Could you check a few things on this model? Use its own coordinates, in mm. A direction names the side the tool comes from. Coordinates: 2 decimals unless noted, no trailing zeros. Loops run counter-clockwise (first coordinate to the right, second up) from the corner with the lowest first, then second, coordinate; pieces in that order, holes last. Notation, with made-up numbers: (55.5, -39.75) -> (87.5, -39.75) arc R28 ccw to (87.5, -8.75) -> close; hole circle Ø2 at (17, 38.25). An arc over 180 degrees is marked (long way). One line per question, with ' | ' between items.
from build123d import *

# Parameters (mm, degrees)
F1_DEPTH = 4
F0_R     = 1.5
F2_DEPTH = 1


with BuildPart() as f1:
    # F0 (on Top) → F1 (new body)
    with BuildSketch(Plane.XY):
        Polygon((11.5, 35.8), (-11.5, 35.8), (-11.5, -35.8), (11.5, -35.8), (11.5, -34.45), (-10.15, -34.45), (-10.15, 34.45), (11.5, 34.45), align=None)
    extrude(amount=F1_DEPTH)

    # F0 (on Top) → F2 (join)
    with BuildSketch(Plane.XY):
        Polygon((11.5, 5), (11.5, 34.45), (-10.15, 34.45), (-10.15, -34.45), (11.5, -34.45), (11.5, -5), (18.5, -5), (18.5, 5), align=None)
        with Locations((15, 0)):
            Circle(F0_R, mode=Mode.SUBTRACT)
    extrude(amount=F2_DEPTH)


solid = f1.part
1) We'd pull the mould along X, two halves only. Please class faces 4 (the face through (-10.15, 0, 2)), 5 (the face through (0, 35.8, 2)), 6 (the face through (13.5, 0.07, 0.49)): pulls with the +X half, pulls with the -X half, needs draft (parallel to the pull), parting line crosses it, or undercut.
Data:
face 4: pulls with the +X half | face 5: needs draft | face 6: undercut
2) On a 3-axis mill with a long thin cutter (end or side, diameter ignored), from which of +Z, -Z, +X, -X, +Y, -Y can I reach the whole of each face in a straight line? I mean faces 1 (the face through (11.5, 21.5, 0.7)), 2 (the face through (11.5, -21.6, 0.8)), 3 (the face through (1, -34.45, 2)). Say none if no direction works.
Data:
face 1: +Z, -Z, +X, +Y | face 2: +Z, -Z, +X, -Y | face 3: +Z, +X
3) I need wall thicknesses on line 1 along Y through (x, z) = (15, 0.8); line 2 along Y through (x, z) = (-1.75, 2.9); line 3 along Z through (x, y) = (-1, -22.5). Which ranges of each line are inside material? Lowest first, please. Write a range as from..to.
Data:
line 1: -5..-1.5, 1.5..5 | line 2: -35.8..-34.45, 34.45..35.8 | line 3: 0..1
4) If we section it at B-B on x = 15: Please give me the cut outline in (y, z).
Data:
outline: (-5, 0) -> (-1.5, 0) -> (-1.5, 1) -> (-5, 1) -> close; (1.5, 0) -> (5, 0) -> (5, 1) -> (1.5, 1) -> close
5) If we section it at C-C on x = 7: Please give me the cut outline in (y, z), and give its area (3 significant figures).
Data:
outline: (-35.8, 0) -> (35.8, 0) -> (35.8, 4) -> (34.45, 4) -> (34.45, 1) -> (-34.45, 1) -> (-34.45, 4) -> (-35.8, 4) -> close | area: 79.7 mm²
6) I'm going to push flat-ended pins straight in: pin 1 Ø2.5 at (x, y) = (15, 0) entering from -Z; pin 2 Ø0.5 at (x, z) = (14, 0.5) entering from -Y; pin 3 Ø0.9 at (y, z) = (-4.5, 3) entering from +X; pin 4 Ø0.8 at (x, z) = (16.5, 0.5) entering from +Y. Where does each tip first touch, or does it pass through?
Data:
pin 1: through | pin 2: y = -5 | pin 3: x = -10.15 | pin 4: y = 5
7) If we section it at D-D on z = 1.65: Please give me the cut outline in (x, y), and give its area (3 significant figures).
Data:
outline: (-11.5, -35.8) -> (11.5, -35.8) -> (11.5, -34.45) -> (-10.15, -34.45) -> (-10.15, 34.45) -> (11.5, 34.45) -> (11.5, 35.8) -> (-11.5, 35.8) -> close | area: 155 mm²
8) If we section it at A-A on y = 0: Please give me the cut outline in (x, z).
Data:
outline: (-11.5, 0) -> (13.5, 0) -> (13.5, 1) -> (-10.15, 1) -> (-10.15, 4) -> (-11.5, 4) -> close; (16.5, 0) -> (18.5, 0) -> (18.5, 1) -> (16.5, 1) -> close
